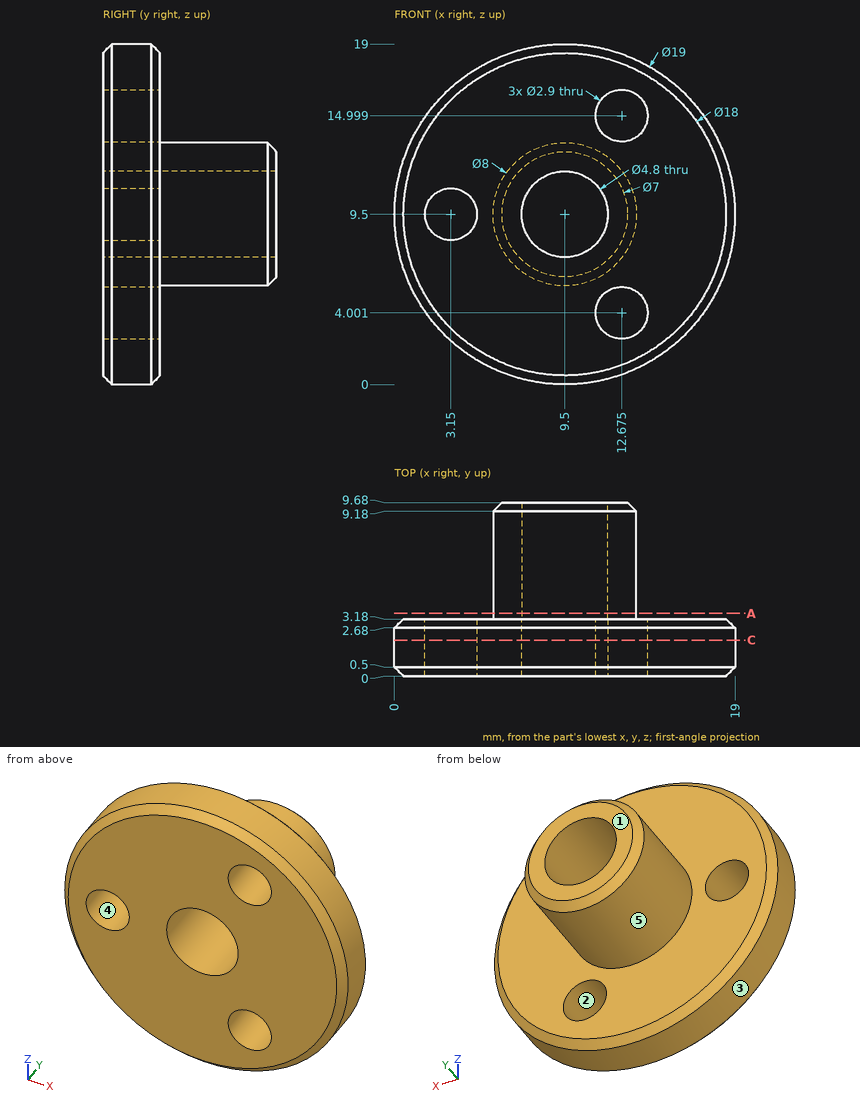
Design review of the part shown in the three views and the two pictorial views. Dimensions are in mm from the part's minimum x, y and z. A direction names the side the tool comes from. Coordinates: 2 decimals unless noted, no trailing zeros. Order: outer loops, then holes, each group sorted by start corner. A loop starts at its lowest first (then second) coordinate and runs counter-clockwise, first axis right, second up.
Item 1: The part is to be moulded in two halves that separate along X. For the marked faces 1, 2 and 3, say which applies: pulls with the +X half, pulls with the -X half, needs draft (parallel to the pull), parting line crosses it, or undercut.
Item 2: Take a section at C-C, the plane y = 2. Count the separate pieces of the cut face and the enclosed holes in it, then the cut area to 3 significant figures.
Item 3: Take a section at A-A, the plane y = 3.5. Write out the cut boundary in (x, z).
Item 4: For the marked faces 4 and 5, list the 3-axis set-ups (+Z, -Z, +X, -X, +Y, -Y) from which the entire face can be reached by the end or side of a thin tool; tool diameter is ignored.
Item 5: For pin 1 Ø4.5 at (x, z) = (12.68, 4) entering from +Y; pin 2 Ø5 at (x, y) = (12.5, 8.5) entering from -Z; pin 3 Ø1.5 at (y, z) = (5, 5.5) entering from -X, all flat-tipped, find the tip position at first contact; note any pin that passes through.
Item 6: For line 1 (Z direction, x = 9.5, y = 7.75); line 2 (Y direction, x = 4.25, z = 7.75), list the stretches that pass through material, from the lowest coordinate up.
The answers:
1. face 1: needs draft
1. face 2: undercut
1. face 3: parting line crosses it
2. separate pieces: 1
2. enclosed holes: 4
2. area: 246 mm2
3. outline: circle Ø8 at (9.5, 9.5); hole circle Ø4.8 at (9.5, 9.5)
4. face 4: +Y, -Y
4. face 5: +Y
5. pin 1: stops at y = 3.18
5. pin 2: stops at z = 5.53
5. pin 3: stops at x = 7.17
6. line 1: z = 5.5 to 7.1, 11.9 to 13.5
6. line 2: y = 0 to 3.18
